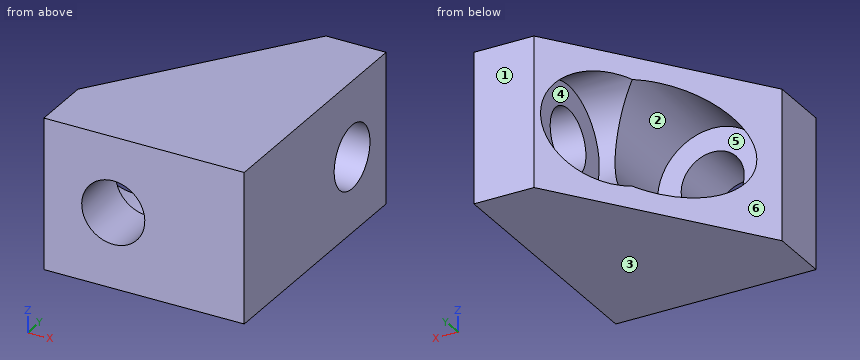
```python
from build123d import *

# Parameters (mm, degrees)
BOSS_EXTRUDE2_DEPTH = 15
SKETCH4_R           = 3.15
CUT_EXTRUDE1_DEPTH  = 46.776415929
SKETCH4_3_R         = 5.5
SKETCH4_3_R_2       = 3.15
CUT_EXTRUDE2_DEPTH  = 14
SKETCH6_R           = 3.15
CUT_EXTRUDE3_DEPTH  = 49.171363436
SKETCH6_3_R         = 5.5
SKETCH6_3_R_2       = 3.15
CUT_EXTRUDE4_DEPTH  = 32.34684153


with BuildPart() as part:
    # Sketch3 → Boss-Extrude2 (new body)
    with BuildSketch(Plane.XY):
        Polygon((18.34684153, 0), (38.34684153, 0), (38.34684153, 25), (32.34684153, 25), (18.34684153, 6), align=None)
    extrude(amount=BOSS_EXTRUDE2_DEPTH)

    # Sketch4 → Cut-Extrude1 (cut, through all)
    with BuildSketch(Plane(origin=(0, 20, 0), x_dir=(1, 0, 0), z_dir=(0, 1, 0))):
        with Locations(Location((25.27040153, -7.5, 0), (0, 0, 270))):
            Circle(SKETCH4_R)
    extrude(amount=-CUT_EXTRUDE1_DEPTH, mode=Mode.SUBTRACT)

    # Sketch4<3> → Cut-Extrude2 (cut)
    with BuildSketch(Plane(origin=(0, 20, 0), x_dir=(1, 0, 0), z_dir=(0, 1, 0))):
        with Locations(Location((25.27040153, -7.5, 0), (0, 0, 270))):
            Circle(SKETCH4_3_R)
        with Locations(Location((25.27040153, -7.5, 0), (0, 0, 270))):
            Circle(SKETCH4_3_R_2, mode=Mode.SUBTRACT)
    extrude(amount=-CUT_EXTRUDE2_DEPTH, mode=Mode.SUBTRACT)

    # Sketch6 → Cut-Extrude3 (cut, through all)
    with BuildSketch(Plane(origin=(0, 0, 0), x_dir=(0, 0, -1), z_dir=(1, 0, 0))):
        with Locations(Location((-7.5, 19, 0), (0, 0, 161.490595018))):
            Circle(SKETCH6_R)
    extrude(amount=CUT_EXTRUDE3_DEPTH, mode=Mode.SUBTRACT)

    # Sketch6<3> → Cut-Extrude4 (cut)
    with BuildSketch(Plane(origin=(0, 0, 0), x_dir=(0, 0, -1), z_dir=(1, 0, 0))):
        with Locations(Location((-7.5, 19, 0), (0, 0, 180))):
            Circle(SKETCH6_3_R)
        with Locations(Location((-7.5, 19, 0), (0, 0, 180))):
            Circle(SKETCH6_3_R_2, mode=Mode.SUBTRACT)
    extrude(amount=CUT_EXTRUDE4_DEPTH, mode=Mode.SUBTRACT)


solid = part.part
```
Here's how the part is built. I have some questions about the finished solid (model axes, mm). Face numbers are marked on the shaded views. A direction names the side the tool comes from. Coordinates: 2 decimals unless noted, no trailing zeros. Order: outer loops, then holes, each group sorted by start corner. A loop starts at its lowest first (then second) coordinate and runs counter-clockwise, first axis right, second up.
Item 1: If we section it at A-A, the plane z = 10: List the corners of the cut face in (x, y) for me, then the cut area to 3 significant figures.
Response values:
outline: (18.35, 0) - (23.35, 0) - (23.35, 6) - (20.37, 6) - (20.37, 8.75) - (18.35, 6) - close; (27.19, 0) - (38.35, 0) - (38.35, 17.08) - (32.35, 17.08) - (32.35, 14.1) - (30.17, 14.1) - (30.17, 6) - (27.19, 6) - close; (31.54, 23.9) - (32.35, 23.9) - (32.35, 20.92) - (38.35, 20.92) - (38.35, 25) - (32.35, 25) - close
area: 209 mm2
Item 2: If we section it at B-B, the plane z = 1: List the corners of the cut face in (x, y) for me, then the cut area to 3 significant figures.
Response values:
outline: (18.35, 0) - (38.35, 0) - (38.35, 25) - (32.35, 25) - (18.35, 6) - close
area: 367 mm2
Item 3: If we section it at D-D, the plane y = 19: List the corners of the cut face in (x, z) for me.
Response values:
outline: (27.93, 0) - (38.35, 0) - (38.35, 4.35) - (32.35, 4.35) - (32.35, 2) - (27.93, 2) - close; (27.93, 13) - (32.35, 13) - (32.35, 10.65) - (38.35, 10.65) - (38.35, 15) - (27.93, 15) - close
Item 4: I need wall thicknesses on probe 1 along Z at (x, y) = (36, 19); probe 2 along Y at (x, z) = (34.85, 7.5); probe 3 along X at (y, z) = (4.05, 7.5). Which ranges of each line are inside material? Lowest first, please.
Response values:
probe 1: z = 0 to 4.35, 10.65 to 15
probe 2: y = 0 to 15.85, 22.15 to 25
probe 3: x = 18.35 to 22.12, 28.42 to 38.35
Item 5: If we section it at C-C, the plane x = 26.5: List the corners of the cut face in (y, z) for me (3 decimals), then the cut area to 3 significant figures.
Response values:
outline: (0, 0) - (17.065, 0) - (17.065, 2.139) - (6, 2.139) - (6, 4.6) - (0, 4.6) - close; (0, 10.4) - (6, 10.4) - (6, 12.861) - (17.065, 12.861) - (17.065, 15) - (0, 15) - close
area: 103 mm2
Item 6: I'm going to push flat-ended pins straight in: pin 1 Ø2 at (y, z) = (12, 8) entering from -X; pin 2 Ø8 at (x, z) = (26, 4.5) entering from +Y; pin 3 Ø5.5 at (y, z) = (21, 8.5) entering from -X. Where does each tip first touch, or does it pass through?
Response values:
pin 1: stops at x = 30.56
pin 2: stops at y = 20.98
pin 3: stops at x = 32.35
Item 7: Thinking about a two-plate mould opening in Z: for the marked faces 1, 2 and 3, which applies, pulls with the +Z half, pulls with the -Z half, needs draft (parallel to the pull), parting line crosses it, or undercut?
Response values:
face 1: needs draft
face 2: undercut
face 3: pulls with the -Z half
Item 8: Which directions (+Z, -Z, +X, -X, +Y, -Y) give clear straight access to the entire face, cutting with the end or side of a thin tool? Please do the marked faces 4, 5 and 6.
Response values:
face 4: -X
face 5: +Y
face 6: +Z, -Z, -X, +Y
